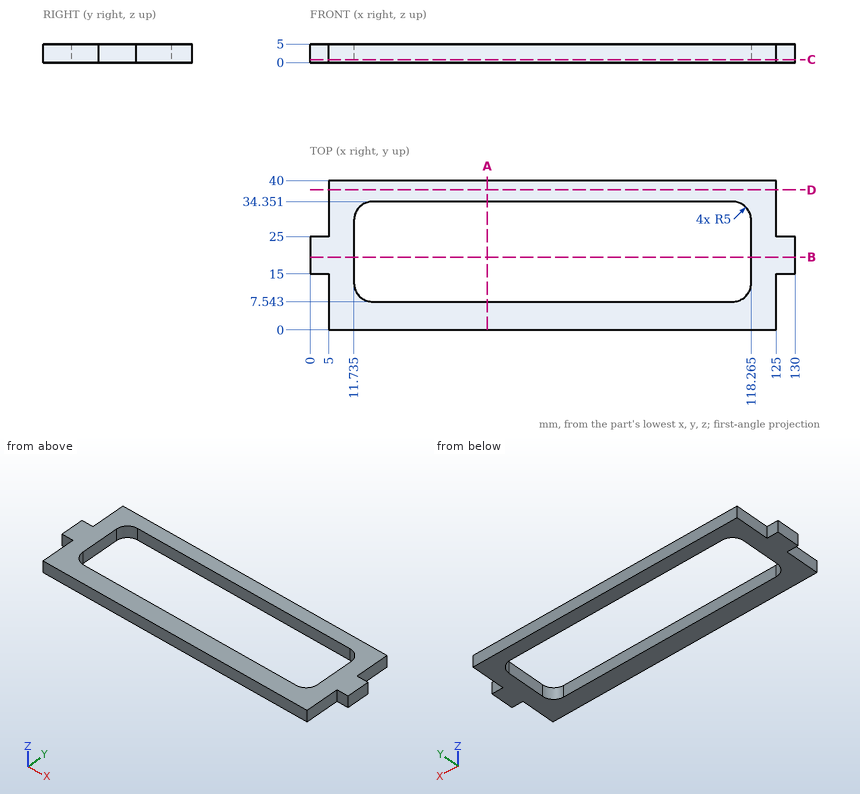
Geometry: see drawing. Coordinates: mm, zero at the bounding-box minimum. Round coordinates to 2 decimals unless told otherwise and drop trailing zeros. Write each loop counter-clockwise with the first axis right and the second up, starting at its lowest first coordinate (ties: lowest second). Pieces come first, ordered by that corner, then holes.
Item 1: Pin query (flat end, axial travel): P1, Ø2.5, axis at y = 5, z = 2.5, coming from the -X side; P2, Ø1.5, axis at x = 127.5, z = 3, coming from the +Y side; P3, Ø1.5, axis at x = 127, z = 2, coming from the -Y side. Return the tip coordinate at first contact, or that it passes through.
Item 2: Section query C-C (z = 0.8). Return loops of the section in (x, y) (1 decimal), plus the area to 3 significant figures.
Item 3: Material intervals for L1, parallel to Y at x = 35.5, z = 2.5; L2, parallel to X at y = 18, z = 2.05 (1 decimal); L3, parallel to X at y = 29, z = 3.6 (1 decimal), sorted ascending.
Item 4: Section query D-D (y = 37.5). Return loops of the section in (x, z).
Item 5: Section query A-A (x = 47.5). Return loops of the section in (y, z).
Item 6: Section query B-B (y = 19.5). Return loops of the section in (x, z) (1 decimal).
Completed:
1. P1: stops at x = 5
1. P2: stops at y = 25
1. P3: stops at y = 15
2. outline: (0, 15) - (5, 15) - (5, 0) - (125, 0) - (125, 15) - (130, 15) - (130, 25) - (125, 25) - (125, 40) - (5, 40) - (5, 25) - (0, 25) - close; hole (11.7, 12.5) arc R5 ccw to (16.7, 7.5) - (113.3, 7.5) arc R5 ccw to (118.3, 12.5) - (118.3, 29.4) arc R5 ccw to (113.3, 34.4) - (16.7, 34.4) arc R5 ccw to (11.7, 29.4) - close
2. area: 2,070 mm2
3. L1: y = 0 to 7.54, 34.35 to 40
3. L2: x = 0 to 11.7, 118.3 to 130
3. L3: x = 5 to 11.7, 118.3 to 125
4. outline: (5, 0) - (125, 0) - (125, 5) - (5, 5) - close
5. outline: (0, 0) - (7.54, 0) - (7.54, 5) - (0, 5) - close; (34.35, 0) - (40, 0) - (40, 5) - (34.35, 5) - close
6. outline: (0, 0) - (11.7, 0) - (11.7, 5) - (0, 5) - close; (118.3, 0) - (130, 0) - (130, 5) - (118.3, 5) - close
